Build history of the part. All positions in model axes, mm. Face numbers are marked on the shaded views. A direction names the side the tool comes from. Give positions to 0.01 mm unless a question says otherwise; leave off trailing zeros. Order: outer loops, then holes, each group sorted by start corner. A loop starts at its lowest first (then second) coordinate and runs counter-clockwise, first axis right, second up. Notation, with made-up numbers: (-26.75, -20.5) - (-7.75, -20.5) arc R18 cw to (-7.75, 4.5) - close; hole circle Ø10 at (-31, -9.5). An arc over 180 degrees is marked (long way). Use a Markdown table: item, result.
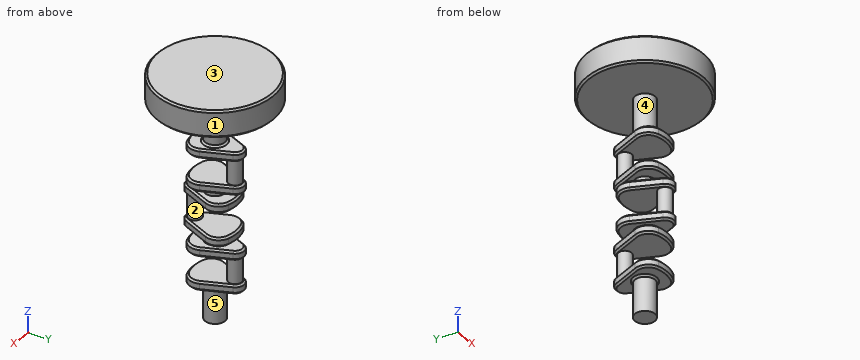
from build123d import *

# Parameters (mm, degrees)
SKETCH1_R             = 9.525
BOSS_EXTRUDE1_DEPTH   = 34.925
BOSS_EXTRUDE2_DEPTH   = 12.7
FILLET1_R             = 19.05
SKETCH3_R             = 14.2875
BOSS_EXTRUDE3_DEPTH   = 9.525
LPATTERN1_COUNT       = 3
LPATTERN1_PITCH       = 69.85
BODY_MOVE_COPY1_ANGLE = 180
LPATTERN2_COUNT       = 2
LPATTERN2_PITCH       = 69.85
SKETCH4_R             = 14.2875
BOSS_EXTRUDE4_DEPTH   = 57.15
BOSS_EXTRUDE5_START   = 50.8
SKETCH5_R             = 14.2875
BOSS_EXTRUDE5_DEPTH   = 50.8
SKETCH6_R             = 83.107085054
BOSS_EXTRUDE6_DEPTH   = 38.1
CHAMFER1_SIZE         = 2.54


with BuildPart() as part:
    # Sketch1 → Boss-Extrude1 (new body)
    with BuildSketch(Plane.XY):
        Circle(SKETCH1_R)
    extrude(amount=-BOSS_EXTRUDE1_DEPTH)

    # Sketch2 → Boss-Extrude2 (add)
    with BuildSketch(Plane(origin=(0, 0, -34.925), x_dir=(-1, 0, 0), z_dir=(0, 0, -1))):
        with BuildLine():
            Line((-11.733270063, 4.860079591), (-33.507418174, -47.707364088))
            ThreePointArc((-33.507418174, -47.707364088), (0, -60.325), (33.507418174, -47.707364088))
            Line((33.507418174, -47.707364088), (11.733270063, 4.860079591))
            ThreePointArc((11.733270063, 4.860079591), (0, 12.7), (-11.733270063, 4.860079591))
        make_face()
    extrude(amount=BOSS_EXTRUDE2_DEPTH)

    # Fillet1
    fillet1_edges = [part.edges().sort_by_distance(p)[0] for p in [
        (33.507418174, -47.707364088, -41.275),
        (-33.507418174, -47.707364088, -41.275),
    ]]
    fillet(fillet1_edges, radius=FILLET1_R)

    # Mirror2: part across plane


with BuildPart() as part_1:
    add(part.part)
    add(part.part.mirror(Plane.XY.offset(-17.4625)))


with BuildPart() as body_2:
    # Sketch3 → Boss-Extrude3 (new body)
    with BuildSketch(Plane(origin=(0, 0, -47.625), x_dir=(-1, 0, 0), z_dir=(0, 0, -1))):
        with Locations(Location((0, -28.486474017, 0), (0, 0, 180))):
            Circle(SKETCH3_R)
    boss_extrude3 = extrude(amount=BOSS_EXTRUDE3_DEPTH)


with BuildPart() as lpattern1_1:
    # LPattern1: pattern copy
    add(part_1.part.moved(Location(Vector(0, 0, -1) * (1 * LPATTERN1_PITCH))))


with BuildPart() as lpattern1_2:
    # LPattern1: pattern copy
    add(part_1.part.moved(Location(Vector(0, 0, -1) * (2 * LPATTERN1_PITCH))))

    # Sketch5 → Boss-Extrude5 (add)
    with BuildSketch(Plane(origin=(0, 0, -187.325), x_dir=(-1, 0, 0), z_dir=(0, 0, -1)).offset(BOSS_EXTRUDE5_START)):
        with Locations(Location((0, -28.486474017, 0), (0, 0, 180))):
            Circle(SKETCH5_R)
    extrude(amount=-BOSS_EXTRUDE5_DEPTH)


with BuildPart() as lpattern1_1_1:
    # Body-Move_Copy1: moved
    add(lpattern1_1.part.rotate(Axis((0, -28.486474017, 0), (0, 0, 1)), BODY_MOVE_COPY1_ANGLE))


with BuildPart() as lpattern2_1:
    # LPattern2: Boss-Extrude3 ×2
    with Locations(*[(0, 0, -i * LPATTERN2_PITCH) for i in range(1, LPATTERN2_COUNT)]):
        add(boss_extrude3)


with BuildPart() as part_2:
    add(part_1.part)

    # Sketch4 → Boss-Extrude4 (add)
    with BuildSketch(Plane.XY.offset(12.7)):
        with Locations((0, -28.486474017)):
            Circle(SKETCH4_R)
    extrude(amount=BOSS_EXTRUDE4_DEPTH)

    # Sketch6 → Boss-Extrude6 (add)
    with BuildSketch(Plane.XY.offset(69.85)):
        with Locations(Location((0, -28.486474017, 0), (0, 0, 180))):
            Circle(SKETCH6_R)
    extrude(amount=BOSS_EXTRUDE6_DEPTH)


with BuildPart() as body_2_1:
    add(body_2.part)

    # Combine1: union LPattern1_1, LPattern2_1, LPattern1_2, part
    add(lpattern1_1_1.part)
    add(lpattern2_1.part)
    add(lpattern1_2.part)
    add(part_2.part)

    # Chamfer1
    chamfer1_edges = [body_2_1.edges().sort_by_distance(p)[0] for p in [
        (0, -69.672948033, -104.775),
        (-19.470080331, -43.154715345, -104.775),
        (0, 3.352051967, -104.775),
        (19.470080331, -43.154715345, -104.775),
        (-19.470080331, -43.154715345, -117.475),
        (-26.88006293, -9.152399421, -117.475),
        (0, 3.352051967, -117.475),
        (26.88006293, -9.152399421, -117.475),
        (19.470080331, -43.154715345, -117.475),
        (0, -69.672948033, -117.475),
        (-26.88006293, -9.152399421, -104.775),
        (26.88006293, -9.152399421, -104.775),
        (0, -69.672948033, -57.15),
        (-19.470080331, -43.154715345, -57.15),
        (0, 3.352051967, -57.15),
        (19.470080331, -43.154715345, -57.15),
        (0, 3.352051967, -69.85),
        (19.470080331, -43.154715345, -69.85),
        (0, -69.672948033, -69.85),
        (-19.470080331, -43.154715345, -69.85),
        (-26.88006293, -9.152399421, -57.15),
        (-26.88006293, -9.152399421, -69.85),
        (26.88006293, -9.152399421, -57.15),
        (26.88006293, -9.152399421, -69.85),
        (0, 12.7, -174.625),
        (19.470080331, -13.818232688, -174.625),
        (0, -60.325, -174.625),
        (-19.470080331, -13.818232688, -174.625),
        (19.470080331, -13.818232688, -187.325),
        (26.88006293, -47.820548612, -187.325),
        (0, -60.325, -187.325),
        (-26.88006293, -47.820548612, -187.325),
        (-19.470080331, -13.818232688, -187.325),
        (0, 12.7, -187.325),
        (26.88006293, -47.820548612, -174.625),
        (-26.88006293, -47.820548612, -174.625),
        (0, 12.7, -127),
        (19.470080331, -13.818232688, -127),
        (0, -60.325, -127),
        (-19.470080331, -13.818232688, -127),
        (0, -60.325, -139.7),
        (-19.470080331, -13.818232688, -139.7),
        (0, 12.7, -139.7),
        (19.470080331, -13.818232688, -139.7),
        (26.88006293, -47.820548612, -127),
        (26.88006293, -47.820548612, -139.7),
        (-26.88006293, -47.820548612, -127),
        (-26.88006293, -47.820548612, -139.7),
        (-14.2875, -28.486474017, -187.325),
        (0, 12.7, -34.925),
        (19.470080331, -13.818232688, -34.925),
        (0, -60.325, -34.925),
        (-19.470080331, -13.818232688, -34.925),
        (19.470080331, -13.818232688, -47.625),
        (26.88006293, -47.820548612, -47.625),
        (0, -60.325, -47.625),
        (-26.88006293, -47.820548612, -47.625),
        (-19.470080331, -13.818232688, -47.625),
        (0, 12.7, -47.625),
        (26.88006293, -47.820548612, -34.925),
        (-26.88006293, -47.820548612, -34.925),
        (0, 12.7, 12.7),
        (19.470080331, -13.818232688, 12.7),
        (0, -60.325, 12.7),
        (-19.470080331, -13.818232688, 12.7),
        (0, -60.325, 0),
        (-19.470080331, -13.818232688, 0),
        (0, 12.7, 0),
        (19.470080331, -13.818232688, 0),
        (26.88006293, -47.820548612, 12.7),
        (26.88006293, -47.820548612, 0),
        (-26.88006293, -47.820548612, 12.7),
        (-26.88006293, -47.820548612, 0),
        (-14.2875, -28.486474017, 12.7),
        (83.107085054, -28.486474017, 69.85),
        (83.107085054, -28.486474017, 107.95),
    ]]
    chamfer(chamfer1_edges, length=CHAMFER1_SIZE)


solid = body_2_1.part
1) Tool access for the marked faces 1 and 2: list every direction of +Z, -Z, +X, -X, +Y, -Y with a clear straight run to the whole face (end or side of a thin tool).
Computed:
| item | result |
|---|---|
| face 1 | +Z, -Z |
| face 2 | none |
2) Wall check: line 1 (Z direction, x = -11.5, y = -33.5) (3 decimals); line 2 (Z direction, x = -28, y = -21.5); line 3 (Z direction, x = 32, y = -4.5). Give the ranges that are in metal, low to high. Write a range as from..to.
Computed:
| item | result |
|---|---|
| line 1 | z = -238.125..-174.625, -139.7..-104.775, -69.85..-34.925, 0..107.95 |
| line 2 | z = -115.09..-107.16, -67.47..-59.53, 69.85..107.95 |
| line 3 | z = 69.85..107.95 |
3) Slice it at B-B (z = -200). Write the cut outline in (x, y) (1 decimal), and give its area (3 significant figures).
Computed:
| item | result |
|---|---|
| outline | circle Ø28.6 at (0, -28.5) |
| area | 641 mm² |
4) Two-plate mould, pull along Z, no slides. Class the marked faces 3, 4 and 5: +Z half, -Z half, draft (parallel to the pull), parting line (faces both ways), or undercut.
Computed:
| item | result |
|---|---|
| face 3 | +Z half |
| face 4 | undercut |
| face 5 | draft |
5) Slice it at A-A (z = -15). Write the cut outline in (x, y) (3 decimals), and give its area (3 significant figures).
Computed:
| item | result |
|---|---|
| outline | circle Ø19.05 at (0, 0) |
| area | 285 mm² |
6) Pin check, flat tips, straight feed: P1, Ø8, axis at y = 0.5, z = -163, coming from the -X side (3 decimals); P2, Ø12, axis at x = -21.5, z = 10.5, coming from the +Y side. Stop position of each tip, or through.
Computed:
| item | result |
|---|---|
| P1 | stops at x = -9.525 |
| P2 | stops at y = -4.26 |
